Build history of the part. All positions in model axes, mm. A direction names the side the tool comes from. Give positions to 0.01 mm unless a question says otherwise; leave off trailing zeros. Loops run counter-clockwise (first coordinate to the right, second up) from the corner with the lowest first, then second, coordinate; pieces in that order, holes last. Notation, with made-up numbers: (-7, 19) - (41, 19) arc R13 ccw to (41, 38) - close; hole circle Ø2 at (73, 68.5). An arc over 180 degrees is marked (long way). Return JSON: item names as keys, results as strings. Group by question number.
1) Slice it at D-D (z = 3.85). Count the separate pieces of the cut face and the enclosed holes in it, and give its area (3 significant figures).
2) Mould opens along X. For faces 1 (the face through (-33, 60, 2)), 2 (the face through (-45, -25, 2)), 3 (the face through (29.6, -32, 2.5)) say: released by +X, released by -X, zero draft, split by the parting line, or undercut.
3) 3-axis set-ups, long thin cutter, end or side, ignore diameter. For faces 4 (the face through (-48, 30, 2)), 5 (the face through (45, 45, 2)), 6 (the face through (33, -40, 2)), 7 (the face through (-32, -40, 2)): which of +Z, -Z, +X, -X, +Y, -Y reach the whole face in a straight line?
4) Slice it at A-A (y = 0). List the corners of the cut face in (x, z).
5) Drop flat-ended pins along their axis: pin 1 (1.5 mm diameter, centred on y = -17, z = 1.5, fed in from -X); pin 2 (3 mm diameter, centred on y = -32.5, z = 2, fed in from +X); pin 3 (2 mm diameter, centred on x = 38.5, z = 4, fed in from -Y). Give the stop position or say it passes through.
6) Slice it at B-B (x = 36.06). List the corners of the cut face in (y, z), and give its area (3 significant figures).
7) Slice it at C-C (y = -36.06). List the corners of the cut face in (x, z), and give its area (3 significant figures).
8) Drill centre lines: probe 1 along Y at (x, z) = (0, 3.65); probe 2 along Y at (x, z) = (37, 2.6); probe 3 along Y at (x, z) = (-28.5, 3.2). Where is each one in solid material? Low to high. Write a range as from..to.
```python
from build123d import *

# Parameters (mm, degrees)
SKETCH1_R           = 2
SKETCH1_R_2         = 32.5
BOSS_EXTRUDE1_DEPTH = 5


with BuildPart() as part:
    # Sketch1 → Boss-Extrude1 (new body)
    with BuildSketch(Plane.XY):
        Polygon((45, -40), (20, -40), (20, -45), (-20, -45), (-20, -40), (-45, -40), (-45, -10), (-50, -10), (-50, 30), (-45, 30), (-45, 60), (-20, 60), (-20, 65), (20, 65), (20, 60), (45, 60), (45, 30), (50, 30), (50, -10), (45, -10), align=None)
        with Locations((-36.06, 36.06)):
            Circle(SKETCH1_R, mode=Mode.SUBTRACT)
        with Locations((36.06, 36.06)):
            Circle(SKETCH1_R, mode=Mode.SUBTRACT)
        with Locations((36.06, -36.06)):
            Circle(SKETCH1_R, mode=Mode.SUBTRACT)
        with Locations((-36.06, -36.06)):
            Circle(SKETCH1_R, mode=Mode.SUBTRACT)
        Circle(SKETCH1_R_2, mode=Mode.SUBTRACT)
        with Locations((-30.0520382, 30.0520382)):
            Circle(SKETCH1_R, mode=Mode.SUBTRACT)
        with Locations((30.0520382, 30.0520382)):
            Circle(SKETCH1_R, mode=Mode.SUBTRACT)
        with Locations((30.0520382, -30.0520382)):
            Circle(SKETCH1_R, mode=Mode.SUBTRACT)
        with Locations((-30.0520382, -30.0520382)):
            Circle(SKETCH1_R, mode=Mode.SUBTRACT)
    extrude(amount=BOSS_EXTRUDE1_DEPTH)


solid = part.part
```
Results:
{
 "1": {"separate pieces": "1", "enclosed holes": "9", "area": "6,380 mm2"},
 "2": {"face 1": "zero draft", "face 2": "released by -X", "face 3": "undercut"},
 "3": {"face 4": "+Z, -Z, -X, +Y", "face 5": "+Z, -Z, +X, +Y", "face 6": "+Z, -Z, +X, -Y", "face 7": "+Z, -Z, -X, -Y"},
 "4": {"outline": "(-50, 0) - (-32.5, 0) - (-32.5, 5) - (-50, 5) - close; (32.5, 0) - (50, 0) - (50, 5) - (32.5, 5) - close"},
 "5": {"pin 1": "x = -45", "pin 2": "x = 45", "pin 3": "y = -40"},
 "6": {"outline": "(-40, 0) - (-38.06, 0) - (-38.06, 5) - (-40, 5) - close; (-34.06, 0) - (34.06, 0) - (34.06, 5) - (-34.06, 5) - close; (38.06, 0) - (60, 0) - (60, 5) - (38.06, 5) - close", "area": "460 mm2"},
 "7": {"outline": "(-45, 0) - (-38.06, 0) - (-38.06, 5) - (-45, 5) - close; (-34.06, 0) - (34.06, 0) - (34.06, 5) - (-34.06, 5) - close; (38.06, 0) - (45, 0) - (45, 5) - (38.06, 5) - close", "area": "410 mm2"},
 "8": {"probe 1": "-45..-32.5, 32.5..65", "probe 2": "-40..-37.83, -34.29..34.29, 37.83..60", "probe 3": "-40..-31.31, -28.79..-15.62, 15.62..28.79, 31.31..60"}
}
